```python
from build123d import *

# Parameters (mm, degrees)
F0_W = 0.775582
F0_H = 0.396875


with BuildPart() as f1:
    # F0 (on Front) → F1 (revolve)
    with BuildSketch(Plane.XZ):
        Polygon((-2.844283, 0), (-2.38125, 0), (-2.38125, 1.190625), (-2.844283, 1.074867), align=None)
        Polygon((-2.844283, 1.074867), (-2.38125, 1.190625), (-2.38125, 1.5875), (-7.9375, 0), (-7.14375, 0), align=None)
        with Locations((-1.993459, 1.389063)):
            Rectangle(F0_W, F0_H)
        Polygon((-2.38125, 1.5875), (-1.605668, 1.5875), (-1.5875, 3.175), (-2.38125, 3.175), align=None)
    revolve(axis=Axis((0, 0, 0.79375), (0, 0, 1)))


solid = f1.part
```
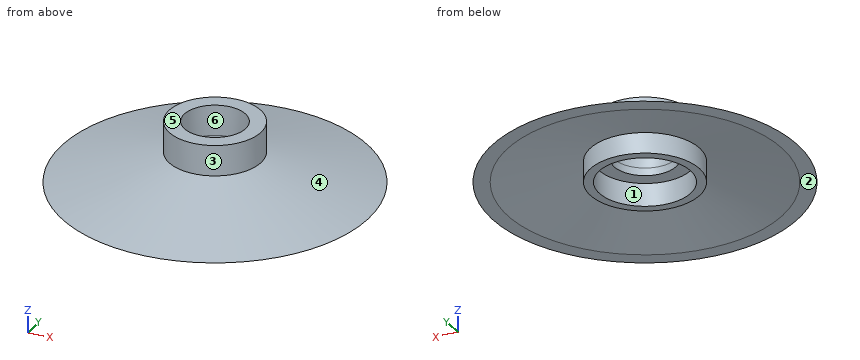
Geometry: final body of the model. Coordinates: model frame, mm. Face numbers are marked on the shaded views. A direction names the side the tool comes from. Coordinates: 2 decimals unless noted, no trailing zeros. Order: outer loops, then holes, each group sorted by start corner. A loop starts at its lowest first (then second) coordinate and runs counter-clockwise, first axis right, second up. Notation, with made-up numbers: (79.25, -28.75) -> (131.25, -28.75) arc R26 cw to (131.25, -1.75) -> close; hole circle Ø8 at (26, 80). An arc over 180 degrees is marked (long way). Answer in a Markdown table with one row per item.
Item 1: Draft query along X for the marked faces 4, 5 and 6. Return one class per face: released by +X, released by -X, zero draft, split by the parting line, or undercut.
Return value:
| item | result |
|---|---|
| face 4 | split by the parting line |
| face 5 | zero draft |
| face 6 | undercut |
Item 2: Ray query, L1, parallel to Y at x = 1, z = 1.75; L2, parallel to Z at x = 1.75, y = -0.75 (3 decimals); L3, parallel to X at y = -2, z = 1.65. Return the intervals inside material, ascending.
Return value:
| item | result |
|---|---|
| L1 | y = -2.16 to -1.25, 1.25 to 2.16 |
| L2 | z = 1.191 to 3.175 |
| L3 | x = -1.29 to 1.29 |
Item 3: Access query for the marked faces 1, 2 and 3. Directions: +Z, -Z, +X, -X, +Y, -Y. A direction counts if a zero-diameter tool reaches every point of the face in a straight line with its end or side. Return the directions, or none.
Return value:
| item | result |
|---|---|
| face 1 | -Z |
| face 2 | -Z, +X, -X, +Y, -Y |
| face 3 | +Z |
Item 4: Section A-A on z = 0.7. Output: boundary loops of the cut face in (x, y) (1 decimal), plus the area to 3 significant figures.
Return value:
| item | result |
|---|---|
| outline | circle Ø11 at (0, 0); circle Ø5.7 at (0, 0); hole circle Ø8.7 at (0, 0); hole circle Ø4.8 at (0, 0) |
| area | 42.9 mm² |
Item 5: Section B-B on z = 2.55. Output: boundary loops of the cut face in (x, y), plus the area to 3 significant figures.
Return value:
| item | result |
|---|---|
| outline | circle Ø4.76 at (0, 0); hole circle Ø3.19 at (0, 0) |
| area | 9.83 mm² |
